Part model, mm, in its own coordinate system. A direction names the side the tool comes from. Round coordinates to 2 decimals unless told otherwise and drop trailing zeros. Order: outer loops, then holes, each group sorted by start corner. A loop starts at its lowest first (then second) coordinate and runs counter-clockwise, first axis right, second up. Notation, with made-up numbers: (10, -35.75) - (33, -35.75) arc R25 ccw to (33, -23.75) - close; hole circle Ø2 at (87, 46.5). An arc over 180 degrees is marked (long way). Return JSON: item names as keys, results as strings. Group by question number.
Item 1: Saw through at C-C on y = 21.5. List the corners of the cut face in (x, z).
Item 2: Drop flat-ended pins along their axis: pin 1 (6 mm diameter, centred on y = 26, z = 0.5, fed in from +X); pin 2 (1.5 mm diameter, centred on y = 5.5, z = 14, fed in from -X); pin 3 (1.5 mm diameter, centred on y = 35, z = -15, fed in from -X). Give the stop position or say it passes through.
Item 3: Saw through at D-D on y = 3. List the corners of the cut face in (x, z).
Item 4: Probe probe 1 along Z at (x, y) = (-128.15, 20); probe 2 along Z at (x, y) = (-125.5, 11.5); probe 3 along Y at (x, z) = (-128.1, 0). List the from-to ranges inside material, lowest first.
Item 5: Saw through at B-B on x = -124.5. List the corners of the cut face in (y, z), and give its area (3 significant figures).
Item 6: Tool access for faces 5 (the face through (-125.424, 7.163, 2.851)), 6 (the face through (-129.152, 33.817, -12.678)), 7 (the face through (-128.708, 25.453, 0.716)): list every direction of +Z, -Z, +X, -X, +Y, -Y with a clear straight run to the whole face (end or side of a thin tool).
Item 7: Saw through at A-A on z = 0. List the corners of the cut face in (x, y), and give its area (3 significant figures).
Item 8: Two-plate mould, pull along Y, no slides. Class faces 1 (the face through (-129, 6, -14)), 2 (the face through (-126, 20, 20)), 3 (the face through (-127, 0, 0)), 4 (the face through (-129.152, 5.663, 12.655)): released by +Y, released by -Y, zero draft, split by the parting line, or undercut.
Autodesk Inventor part; units mm, degrees
ref_plane "Work Plane1" through (-130, 0, 0) normal (1, 0, 0) x (0, 1, 0)
ref_plane "XZ Plane" through (0, 0, 0) normal (0, 1, 0) x (-1, 0, 0)
ref_plane "XY Plane" through (0, 0, 0) normal (0, 0, 1) x (1, 0, 0)
sketch "Sketch1" plane through (0, 0, 0) normal (0, 1, 0) x (-1, 0, 0)
  arc A0 (128.4523, -20) -> (128.4523, 20) centre (0, 0) ccw
  line L0 (128.4523, 20) -> (123.4523, 20)
  line L1 (123.4523, 20) -> (123.4523, -20)
  line L2 (123.4523, -20) -> (128.4523, -20)
  point P0 (123.4523, 0)
  dimension "d0" = 130
  dimension "d1" = 40
  dimension "d2" = 5
extrude "Extrusion1" add sketch "Sketch1" along normal blind 40
sketch "Sketch2" plane through (-123.4523, 0, 20) normal (1, 0, 0) x (0, 0, -1)
  circle A0 centre (20, 20) radius 13.15
  line L0 (0, 0) -> (0, 40)
  line L1 (0, 0) -> (40, 0)
  point P0 (20, 0)
  point P1 (0, 20)
  point P2 (20, 0)
  dimension "d5" = 26.3
extrude "Extrusion2" cut sketch "Sketch2" against normal blind 4
sketch "Sketch3" plane through (-127.4523, 20, 0) normal (1, 0, 0) x (0, 0, -1)
  circle A0 centre (0, 0) radius 5.5
  point P0 (0, -20)
  dimension "d8" = 11
extrude "Extrusion3" cut sketch "Sketch3" against normal through all
ref_plane "Work Plane1" through (-130, 0, 0) normal (1, 0, 0) x (0, 1, 0)
sketch "Sketch4" plane through (-130, 0, 0) normal (1, 0, 0) x (0, 1, 0)
  circle A0 centre (34.1421, -14.1421) radius 1.5
  circle A1 centre (20, 0) radius 5.5
  circle A2 centre (20, 0) radius 20 construction
  circle A3 centre (34.1421, 14.1421) radius 1.5
  circle A4 centre (5.8579, 14.1421) radius 1.5
  circle A5 centre (5.8579, -14.1421) radius 1.5
  line L0 (20, 0) -> (20, -24.623) construction
  line L1 (20, 0) -> (34.1421, -14.1421) construction
  point P0 (0, 0)
  dimension "d15" = 40
  dimension "d11" = 3
  dimension "d18" = 360
  dimension "d20" = 45
extrude "Extrusion4" cut sketch "Sketch4" along normal blind 1 contours A0 | A3 | A4 | A5
properties part number "shift_fixed_socket" material "Acetal Resin, White"
Filled in:
{
 "1": {"outline": "(-129.89, -5.29) arc R130 ccw to (-128.45, -20) - (-123.45, -20) - (-123.45, -13.06) - (-127.45, -13.06) - (-127.45, -5.29) - close; (-129.89, 5.29) - (-127.45, 5.29) - (-127.45, 13.06) - (-123.45, 13.06) - (-123.45, 20) - (-128.45, 20) arc R130 ccw to start"},
 "2": {"pin 1": "stops at x = -127.45", "pin 2": "stops at x = -129", "pin 3": "stops at x = -129.18"},
 "3": {"outline": "(-128.45, -20) - (-123.45, -20) - (-123.45, 20) - (-128.45, 20) arc R130 ccw to start"},
 "4": {"probe 1": "z = -20 to -5.5, 5.5 to 20", "probe 2": "z = -20 to -10.03, 10.03 to 20", "probe 3": "y = 0 to 14.5, 25.5 to 40"},
 "5": {"outline": "(0, -20) - (40, -20) - (40, 20) - (0, 20) - close; hole circle Ø26.3 at (20, 0)", "area": "1,060 mm^2"},
 "6": {"face 5": "+X", "face 6": "-X", "face 7": "+X, -X"},
 "7": {"outline": "(-130, 0) - (-123.45, 0) - (-123.45, 6.85) - (-127.45, 6.85) - (-127.45, 14.5) - (-130, 14.5) - close; (-130, 25.5) - (-127.45, 25.5) - (-127.45, 33.15) - (-123.45, 33.15) - (-123.45, 40) - (-130, 40) - close", "area": "129 mm^2"},
 "8": {"face 1": "undercut", "face 2": "zero draft", "face 3": "released by -Y", "face 4": "undercut"}
}
